Geometry: final body of the model. Coordinates: model frame, mm. A direction names the side the tool comes from. Give positions to 0.01 mm unless a question says otherwise; leave off trailing zeros. Order: outer loops, then holes, each group sorted by start corner. A loop starts at its lowest first (then second) coordinate and runs counter-clockwise, first axis right, second up. Notation, with made-up numbers: (15.5, -27.5) - (43.5, -27.5) arc R22 ccw to (43.5, -16.5) - close; hole circle Ø3 at (80, 87). An arc over 180 degrees is marked (long way). One line per question, with ' | ' between items. Start each with the question number.
from build123d import *
from build123d.topology import SkipClean

# Parameters (mm, degrees)
FILLET2_R               = 0.25
SKETCH3_R               = 1
BOSS_EXTRUDE1_DEPTH     = 4
CIRPATTERN1_COUNT       = 4
MIRROR1_COPY_1_SKETCH_R = 1
MIRROR1_COPY_1_DEPTH    = 4
MIRROR1_COPY_2_SKETCH_R = 1
MIRROR1_COPY_2_DEPTH    = 4
MIRROR1_COPY_3_SKETCH_R = 1
MIRROR1_COPY_3_DEPTH    = 4
CUT_EXTRUDE1_REACH      = 20.921
SKETCH4_W               = 8
SKETCH4_H               = 8


with BuildPart() as part:
    # Sketch2 → Revolve1 (revolve)
    with BuildSketch(Plane(origin=(0, 0, 0), x_dir=(0, 0, -1), z_dir=(1, 0, 0)), mode=Mode.PRIVATE) as revolve1_sk:
        Polygon((-5, 9), (-5, 0), (0, 0), (0, 7.5), (-3, 7.5), (-3, 9), align=None)
        Polygon((0, 7.5), (0, 0), (5, 0), (5, 9), (3, 9), (3, 7.5), align=None)
    revolve(revolve1_sk.sketch.rotate(Axis((0, 0, 0), (0, 0, -1)), 90), axis=Axis((0, 0, 0), (0, 0, -1)))

    # Fillet2
    fillet2_edges = [part.edges().sort_by_distance(p)[0] for p in [
        (-9, 0, -3),
        (-9, 0, 3),
    ]]
    fillet(fillet2_edges, radius=FILLET2_R)

    # Sketch3 → Boss-Extrude1 (add)
    with BuildSketch(Plane(origin=(0, 0, -5), x_dir=(-1, 0, 0), z_dir=(0, 0, -1))):
        with BuildLine():
            ThreePointArc((2, 8.774964387), (1.006310219, 8.943564152), (0, 9))
            ThreePointArc((0, 9), (-1.006310219, 8.943564152), (-2, 8.774964387))
            ThreePointArc((-2, 8.774964387), (-1.154168213, 8.581704304), (-0.777777778, 7.799968344))
            ThreePointArc((-0.777777778, 7.799968344), (-0.996041818, 7.17635878), (-1.555555556, 6.824972301))
            ThreePointArc((-1.555555556, 6.824972301), (-0.782685726, 6.956105452), (0, 7))
            ThreePointArc((0, 7), (0.782685726, 6.956105452), (1.555555556, 6.824972301))
            ThreePointArc((1.555555556, 6.824972301), (0.802781735, 8.022190567), (2, 8.774964387))
        make_face()
        with Locations((-1.777777778, 7.799968344)):
            Circle(SKETCH3_R)
        with Locations((1.777777778, 7.799968344)):
            Circle(SKETCH3_R)
    boss_extrude1 = extrude(amount=BOSS_EXTRUDE1_DEPTH)

    # CirPattern1: Boss-Extrude1 ×4 about axis
    cirpattern1_axis = Axis((0, 0, 0), (0, 0, 1))
    for i in range(1, CIRPATTERN1_COUNT):
        add(boss_extrude1.rotate(cirpattern1_axis, i * 360 / CIRPATTERN1_COUNT))

    # Mirror1: Boss-Extrude1 across plane
    add(boss_extrude1.mirror(Plane.XY))

    # Mirror1 copy 1 sketch → Mirror1 copy 1 (add)
    with BuildSketch(Plane(origin=(0, 0, 5), x_dir=(0, -1, 0), z_dir=(0, 0, 1))):
        with BuildLine():
            ThreePointArc((2, -8.774964387), (1.006310219, -8.943564152), (0, -9))
            ThreePointArc((0, -9), (-1.006310219, -8.943564152), (-2, -8.774964387))
            ThreePointArc((-2, -8.774964387), (-1.154168213, -8.581704304), (-0.777777778, -7.799968344))
            ThreePointArc((-0.777777778, -7.799968344), (-0.996041818, -7.17635878), (-1.555555556, -6.824972301))
            ThreePointArc((-1.555555556, -6.824972301), (-0.782685726, -6.956105452), (0, -7))
            ThreePointArc((0, -7), (0.782685726, -6.956105452), (1.555555556, -6.824972301))
            ThreePointArc((1.555555556, -6.824972301), (0.802781735, -8.022190567), (2, -8.774964387))
        make_face()
        with Locations((-1.777777778, -7.799968344)):
            Circle(MIRROR1_COPY_1_SKETCH_R)
        with Locations((1.777777778, -7.799968344)):
            Circle(MIRROR1_COPY_1_SKETCH_R)
    extrude(amount=MIRROR1_COPY_1_DEPTH)

    # Mirror1 copy 2 sketch → Mirror1 copy 2 (add)
    with BuildSketch(Plane.XY.offset(5)):
        with BuildLine():
            ThreePointArc((2, -8.774964387), (1.006310219, -8.943564152), (0, -9))
            ThreePointArc((0, -9), (-1.006310219, -8.943564152), (-2, -8.774964387))
            ThreePointArc((-2, -8.774964387), (-1.154168213, -8.581704304), (-0.777777778, -7.799968344))
            ThreePointArc((-0.777777778, -7.799968344), (-0.996041818, -7.17635878), (-1.555555556, -6.824972301))
            ThreePointArc((-1.555555556, -6.824972301), (-0.782685726, -6.956105452), (0, -7))
            ThreePointArc((0, -7), (0.782685726, -6.956105452), (1.555555556, -6.824972301))
            ThreePointArc((1.555555556, -6.824972301), (0.802781735, -8.022190567), (2, -8.774964387))
        make_face()
        with Locations((-1.777777778, -7.799968344)):
            Circle(MIRROR1_COPY_2_SKETCH_R)
        with Locations((1.777777778, -7.799968344)):
            Circle(MIRROR1_COPY_2_SKETCH_R)
    extrude(amount=MIRROR1_COPY_2_DEPTH)

    # Mirror1 copy 3 sketch → Mirror1 copy 3 (add)
    with SkipClean():  # the faces are left unmerged after this step: merging them gives an invalid solid
        with BuildSketch(Plane(origin=(0, 0, 5), x_dir=(0, 1, 0), z_dir=(0, 0, 1))):
            with BuildLine():
                ThreePointArc((2, -8.774964387), (1.006310219, -8.943564152), (0, -9))
                ThreePointArc((0, -9), (-1.006310219, -8.943564152), (-2, -8.774964387))
                ThreePointArc((-2, -8.774964387), (-1.154168213, -8.581704304), (-0.777777778, -7.799968344))
                ThreePointArc((-0.777777778, -7.799968344), (-0.996041818, -7.17635878), (-1.555555556, -6.824972301))
                ThreePointArc((-1.555555556, -6.824972301), (-0.782685726, -6.956105452), (0, -7))
                ThreePointArc((0, -7), (0.782685726, -6.956105452), (1.555555556, -6.824972301))
                ThreePointArc((1.555555556, -6.824972301), (0.802781735, -8.022190567), (2, -8.774964387))
            make_face()
            with Locations((-1.777777778, -7.799968344)):
                Circle(MIRROR1_COPY_3_SKETCH_R)
            with Locations((1.777777778, -7.799968344)):
                Circle(MIRROR1_COPY_3_SKETCH_R)
        extrude(amount=MIRROR1_COPY_3_DEPTH)

    # Sketch4 → Cut-Extrude1 (cut, up to next)
    with BuildSketch(Plane(origin=(0, 0, -5), x_dir=(-1, 0, 0), z_dir=(0, 0, -1)), mode=Mode.PRIVATE) as cut_extrude1_sk1:
        Rectangle(SKETCH4_W, SKETCH4_H)
    cut_extrude1_tool1 = extrude(cut_extrude1_sk1.sketch, amount=-CUT_EXTRUDE1_REACH, mode=Mode.PRIVATE) & part.part
    add(cut_extrude1_tool1.solids().sort_by_distance((0, 0, -5))[0], mode=Mode.SUBTRACT)


solid = part.part
(1) Material intervals for line 1 along Y through (x, z) = (-0.25, 6.25); line 2 along Z through (x, y) = (-4, -6); line 3 along X through (y, z) = (-2, -4.5), sorted ascending. Write a range as from..to.
(2) Cut plane A-A, the plane z = -6.75. Return the cut outline in (x, y), plus the area to 3 significant figures.
(3) Contact query for flat-ended pins moving along their axis: P1, Ø4, axis at x = 4, z = 1.5, coming from the +Y side; P2, Ø3, axis at y = -2.5, z = -3, coming from the -X side; P3, Ø6, axis at x = -5, y = -1.5, coming from the +Z side; P4, Ø1, axis at x = -0.5, y = -6, coming from the +Z side. Output: stop coordinate, or through.
(4) Pull-direction query (Z, two-part tool) for faces 4 (the flat face through (-4, -7, -3)), 5 (the flat face through (0, 8, 9)), 6 (the flat face through (0, -8, -9)), 7 (the flat face through (0, 4, 0)); classes: +Z half, -Z half, draft (parallel to the pull), parting line (faces both ways), or undercut.
(5) Access query for faces 1 (the flat face through (4, 0, 0)), 2 (the flat face through (-8, 0, 9)), 3 (the flat face through (4, -7, 3)). Directions: +Z, -Z, +X, -X, +Y, -Y. A direction counts if a zero-diameter tool reaches every point of the face in a straight line with its end or side. Return the directions, or none.
(6) Cut plane B-B, the plane z = 4.75. Return the cut outline in (x, y).
Results are:
1) line 1: -9..-7, 7..9 | line 2: -5..5 | line 3: -8.77..-4, 4..8.77
2) outline: (-8.77, -2) arc R1 ccw to (-6.82, -1.56) arc R7 cw to (-6.82, 1.56) arc R1 ccw to (-8.77, 2) arc R9 ccw to start; (-2, -8.77) arc R9 ccw to (2, -8.77) arc R1 ccw to (1.56, -6.82) arc R7 cw to (-1.56, -6.82) arc R1 ccw to start; (-2, 8.77) arc R1 ccw to (-1.56, 6.82) arc R7 cw to (1.56, 6.82) arc R1 ccw to (2, 8.77) arc R9 ccw to start; (6.82, -1.56) arc R1 ccw to (8.77, -2) arc R9 ccw to (8.77, 2) arc R1 ccw to (6.82, 1.56) arc R7 cw to start | area: 41.3 mm2
3) P1: y = 8.51 | P2: x = -8.94 | P3: z = 9 | P4: z = 5
4) face 4: undercut | face 5: +Z half | face 6: -Z half | face 7: draft
5) face 1: +Z, -Z | face 2: +Z, +X, -X, +Y, -Y | face 3: none
6) outline: circle Ø18 at (0, 0); hole (-4, -4) - (4, -4) - (4, 4) - (-4, 4) - close
